Autodesk Inventor part; units mm, degrees
ref_plane "YZ Plane" through (0, 0, 0) normal (1, 0, 0) x (0, 1, 0)
ref_plane "XZ Plane" through (0, 0, 0) normal (0, 1, 0) x (-1, 0, 0)
ref_plane "XY Plane" through (0, 0, 0) normal (0, 0, 1) x (1, 0, 0)
sketch "Sketch1" plane through (0, 0, 0) normal (0, 1, 0) x (-1, 0, 0)
  line L0 (195, 302.5) -> (-195, 302.5)
  line L1 (-195, 302.5) -> (-195, -302.5)
  line L2 (-195, -302.5) -> (195, -302.5)
  line L3 (195, -302.5) -> (195, 302.5)
  line L4 (195, 302.5) -> (-195, -302.5) construction
  line L5 (-195, 302.5) -> (195, -302.5) construction
  point P0 (0, 0)
  dimension "d0" = 390
  dimension "d1" = 605
extrude "Extrusion1" add sketch "Sketch1" along normal blind 12
sketch "Sketch2" plane through (0, 12, 0) normal (0, 1, 0) x (1, 0, 0)
  line L0 (-195, 302.5) -> (-195, -302.5)
  line L1 (-195, -302.5) -> (-195, -192.5)
  line L2 (-195, -302.5) -> (-85, -302.5) construction
  line L3 (-195, -192.5) -> (-105, -192.5)
  line L4 (-105, -192.5) -> (-105, -302.5)
  line L5 (-105, -302.5) -> (-195, -302.5)
  point P0 (0, 0)
  dimension "d4" = 110
  dimension "d5" = 90
  dimension "d6" = 90
  dimension "d7" = 90
extrude "Extrusion2" add sketch "Sketch2" along normal blind 80
sketch "Sketch3" plane through (-195, 0, -302.5) normal (-1, 0, 0) x (0, 0, 1)
  line L0 (495, 92) -> (605, 92)
  line L1 (495, 92) -> (550, 92)
  line L2 (550, 92) -> (550, 73)
  line L3 (550, 92) -> (569, 92) construction
  circle A0 centre (550, 73) radius 20
  point P0 (302.5, 0)
  point P1 (543.755, 92)
  point P2 (556.245, 92)
  dimension "d10" = 55
  dimension "d11" = 19
  dimension "d12" = 90
  dimension "d13" = 40
extrude "Extrusion3" cut sketch "Sketch3" against normal blind 110 contours L0 A0 picked at (549.7853, 66.101)
sketch "Sketch4" plane through (-195, 0, -302.5) normal (-1, 0, 0) x (0, 0, 1)
  line L0 (495, 92) -> (543.755, 92)
  line L1 (543.755, 92) -> (533.755, 92)
  line L2 (533.755, 92) -> (537.2905, 88.4645)
  arc A0 (543.755, 92) -> (556.245, 92) centre (550, 73) ccw
  line L3 (537.2905, 88.4645) -> (543.755, 92)
  point P0 (302.5, 0)
  dimension "d16" = 10
  dimension "d17" = 5
  dimension "d18" = 45
extrude "Extrusion4" cut sketch "Sketch4" against normal blind 110
sketch "Sketch5" plane through (-195, 0, -302.5) normal (-1, 0, 0) x (0, 0, 1)
  arc A0 (537.3715, 88.5088) -> (556.245, 92) centre (550, 73) ccw
  line L0 (556.245, 92) -> (566.245, 92)
  line L1 (556.245, 92) -> (605, 92)
  line L2 (556.245, 92) -> (566.245, 92) construction
  line L3 (566.245, 92) -> (562.7095, 88.4645)
  line L4 (562.7095, 88.4645) -> (556.245, 92)
  point P0 (302.5, 0)
  dimension "d21" = 10
  dimension "d22" = 0
  dimension "d23" = 5
  dimension "d24" = 45
extrude "Extrusion5" cut sketch "Sketch5" against normal blind 110
mirror "Mirror1" about plane through (0, 0, 0) normal (0, 0, 1) of "Extrusion2"
sketch "Sketch6" plane through (-105, 12, -302.5) normal (1, 0, 0) x (0, 0, -1)
  line L0 (-110, 80) -> (-55, 80)
  line L1 (0, 80) -> (-110, 80)
  line L2 (-55, 80) -> (-55, 61)
  circle A0 centre (-55, 61) radius 20
  point P0 (-302.5, -12)
  point P1 (-61.245, 80)
  point P2 (-48.755, 80)
  dimension "d27" = 55
  dimension "d28" = 19
  dimension "d29" = 40
extrude "Extrusion6" cut sketch "Sketch6" against normal blind 110 contours L0 L1 A0 picked at (-55.2147, 54.101)
mirror "Mirror2" about plane through (0, 0, 0) normal (1, 0, 0) of "Extrusion2", "Mirror1"
sketch "Sketch7" plane through (195, 0, 302.5) normal (1, 0, 0) x (0, 0, -1)
  arc A0 (543.755, 92) -> (556.245, 92) centre (550, 73) ccw
  circle A1 centre (550, 73) radius 20
  point P0 (302.5, 0)
extrude "Extrusion7" cut sketch "Sketch7" against normal blind 110
sketch "Sketch8" plane through (195, 0, 302.5) normal (1, 0, 0) x (0, 0, -1)
  arc A0 (42.3715, 88.5088) -> (67.6285, 88.5088) centre (55, 73) ccw
  circle A1 centre (55, 73) radius 20
  point P0 (302.5, 0)
  point P1 (67.6285, 88.5088)
extrude "Extrusion8" cut sketch "Sketch8" against normal blind 110
sketch "Sketch9" plane through (195, 0, 302.5) normal (1, 0, 0) x (0, 0, -1)
  line L0 (48.755, 92) -> (38.755, 92)
  line L1 (48.755, 92) -> (0, 92)
  line L2 (38.755, 92) -> (42.3026, 88.4524)
  arc A0 (48.755, 92) -> (61.245, 92) centre (55, 73) ccw
  line L3 (42.3026, 88.4524) -> (48.755, 92)
  point P0 (302.5, 0)
  dimension "d36" = 10
  dimension "d37" = 45
extrude "Extrusion9" cut sketch "Sketch9" against normal blind 110
sketch "Sketch10" plane through (195, 0, 302.5) normal (1, 0, 0) x (0, 0, -1)
  arc A0 (42.3026, 88.4524) -> (61.245, 92) centre (55, 73) ccw
  line L0 (61.245, 92) -> (71.245, 92)
  line L1 (110, 92) -> (61.245, 92)
  line L2 (71.245, 92) -> (67.7095, 88.4645)
  line L3 (67.7095, 88.4645) -> (61.245, 92)
  point P0 (302.5, 0)
  dimension "d40" = 10
  dimension "d41" = 5
  dimension "d42" = 45
extrude "Extrusion10" cut sketch "Sketch10" against normal blind 110
sketch "Sketch11" plane through (195, 0, 302.5) normal (1, 0, 0) x (0, 0, -1)
  line L0 (543.755, 92) -> (495, 92)
  line L1 (543.755, 92) -> (533.755, 92)
  line L2 (533.755, 92) -> (537.2905, 88.4645)
  arc A0 (543.755, 92) -> (556.245, 92) centre (550, 73) ccw
  line L3 (537.2905, 88.4645) -> (543.755, 92)
  point P0 (302.5, 0)
  dimension "d45" = 10
  dimension "d46" = 5
  dimension "d47" = 45
extrude "Extrusion11" cut sketch "Sketch11" against normal blind 110
sketch "Sketch12" plane through (195, 0, 302.5) normal (1, 0, 0) x (0, 0, -1)
  line L0 (556.245, 92) -> (566.245, 92)
  line L1 (605, 92) -> (556.245, 92)
  line L2 (566.245, 92) -> (562.7095, 88.4645)
  arc A0 (537.3715, 88.5088) -> (556.245, 92) centre (550, 73) ccw
  line L3 (562.7095, 88.4645) -> (556.245, 92)
  point P0 (302.5, 0)
  dimension "d50" = 10
  dimension "d51" = 5
  dimension "d52" = 45
extrude "Extrusion12" cut sketch "Sketch12" against normal blind 110
sketch "Sketch13" plane through (-195, 0, -302.5) normal (-1, 0, 0) x (0, 0, 1)
  line L0 (0, 92) -> (48.755, 92)
  line L1 (48.755, 92) -> (38.755, 92)
  line L2 (38.755, 92) -> (42.2905, 88.4645)
  line L3 (42.2905, 88.4645) -> (48.755, 92)
  line L4 (61.245, 92) -> (110, 92)
  line L5 (61.245, 92) -> (71.245, 92)
  line L6 (71.245, 92) -> (67.7095, 88.4645)
  arc A0 (48.755, 92) -> (61.245, 92) centre (55, 73) ccw
  line L7 (67.7095, 88.4645) -> (61.245, 92)
  point P0 (302.5, 0)
  dimension "d55" = 10
  dimension "d56" = 5
  dimension "d57" = 45
  dimension "d58" = 10
  dimension "d59" = 5
  dimension "d60" = 45
extrude "Extrusion13" cut sketch "Sketch13" against normal blind 110
properties part number "Kuka_base"
Source: CAD feature listing. Evaluate the final solid. Frame: model axes, mm. A direction names the side the tool comes from. Round coordinates to 2 decimals unless told otherwise and drop trailing zeros. Loops run counter-clockwise (first coordinate to the right, second up) from the corner with the lowest first, then second, coordinate; pieces in that order, holes last. Notation, with made-up numbers: M -26.75,-2 L 7.25,-2 A20 cw 7.25,16 Z; hole C 52,75.5 d7. An arc over 180 degrees is marked long. Return JSON: item names as keys, results as strings. Group by question number.
1. Section query B-B on z = -247.5. Output: boundary loops of the cut face in (x, y), and give its area (3 significant figures).
2. Mould query, pull axis Z, two halves, no side actions, for faces 1 (the face through (-105, 51, 247)), 2 (the face through (-3, 4, -302.5)), 3 (the face through (-149.37, 53.01, -246.81)). Classes: released by +Z, released by -Z, zero draft, split by the parting line, or undercut.
3. Section query C-C on x = -10.5. Output: boundary loops of the cut face in (y, z), and give its area (3 significant figures).
4. Section query A-A on y = 73. State how many separate pieces and enclosed holes the cut face has, and give its area (3 significant figures).
5. Reachability of faces 4 (the face through (105, 51, -247)), 5 (the face through (149, 92, 212)), 6 (the face through (-151, 51, 192.5)) from +Z, -Z, +X, -X, +Y, -Y: full face, straight path, thin tool, end or side. Return the list, or none.
6. Material intervals for line 1 along Z through (x, y) = (-145, 73); line 2 along Y through (x, z) = (150, 115); line 3 along X through (y, z) = (57.5, 234), sorted ascending. Write a range as from..to.
Checks:
{
 "1": {"outline": "M -195,0 L 195,0 L 195,53 L 105,53 L 105,12 L -105,12 L -105,53 L -195,53 Z", "area": "12,100 mm²"},
 "2": {"face 1": "zero draft", "face 2": "released by -Z", "face 3": "undercut"},
 "3": {"outline": "M 0,-302.5 L 12,-302.5 L 12,302.5 L 0,302.5 Z", "area": "7,260 mm²"},
 "4": {"separate pieces": "8", "enclosed holes": "0", "area": "25,200 mm²"},
 "5": {"face 4": "+Z, -Z, +Y", "face 5": "+Z, -Z, +X, -X, +Y", "face 6": "+X, -X, +Y"},
 "6": {"line 1": "z = -302.5..-267.5, -227.5..-192.5, 192.5..227.5, 267.5..302.5", "line 2": "y = 0..12", "line 3": "x = -195..-105, 105..195"}
}
